Design review of the part built by this model. Coordinates are the model's own, in mm. Face numbers are marked on the shaded views. A direction names the side the tool comes from. Coordinates: 2 decimals unless noted, no trailing zeros. Loops run counter-clockwise (first coordinate to the right, second up) from the corner with the lowest first, then second, coordinate; pieces in that order, holes last.
Q1. Add section A-A on y = 23.5. Give the boundary of the cut face in (x, z).
Q2. Machinability: for the marked faces 1 and 2, which of the approach directions +Z, -Z, +X, -X, +Y, -Y give a long, thin tool a straight path to every point of the face, cutting with its end or side? Answer none if there is none.
Q3. Wall thickness on probe 1 along Y at (x, z) = (70, 10); probe 2 along Y at (x, z) = (83.5, -1); probe 3 along X at (y, z) = (21, 6): over which ranges is each line inside the solid? List them lowest first.
Q4. Add section B-B on y = 4. Give the boundary of the cut face in (x, z), and give its area (3 significant figures).
Q5. For P1, Ø2.5, axis at x = 79.77, z = 7, coming from the +Y side; P2, Ø3.5, axis at x = 70.5, z = -13, coming from the +Y side; P3, Ø5, axis at x = 58, y = 17, coming from the +Z side, all flat-tipped, find the tip position at first contact; note any pin that passes through.
```python
from build123d import *

# Parameters (mm, degrees)
SKETCH5_R             = 1.5
CUT_EXTRUDE1_DEPTH    = 4
SKETCH3_R             = 5
SKETCH3_R_2           = 2.5
BOSS_EXTRUDE3_DEPTH   = 2.5
BODY_MOVE_COPY1_ANGLE = 180
BODY_MOVE_COPY2_ANGLE = 180
BODY_MOVE_COPY3_ANGLE = 90


with BuildPart() as part:
    # Sketch1 → Revolve1 (revolve)
    with BuildSketch(Plane.XY, mode=Mode.PRIVATE) as revolve1_sk:
        with BuildLine():
            Line((33.701320748, 0), (33.701320748, 13.75))
            Line((33.701320748, 13.75), (21.201320748, 13.75))
            Line((21.201320748, 13.75), (8.201320748, 13.75))
            Line((8.201320748, 13.75), (8.201320748, 14.25))
            Line((8.201320748, 14.25), (-11.798679252, 14.25))
            Line((-11.798679252, 14.25), (-11.798679252, 13.75))
            Line((-11.798679252, 13.75), (-15.358679252, 13.75))
            ThreePointArc((-15.358679252, 13.75), (-16.23549166, 13.386812409), (-16.598679252, 12.51))
            Line((-16.598679252, 12.51), (-16.598679252, 12.5))
            Line((-16.598679252, 12.5), (-17.398679252, 12.5))
            Line((-17.398679252, 12.5), (-17.398679252, 15.00458738))
            Line((-17.398679252, 15.00458738), (-40.398679252, 15.00458738))
            Line((-40.398679252, 15.00458738), (-40.398679252, 0))
            Line((-40.398679252, 0), (33.701320748, 0))
        make_face()
    revolve(revolve1_sk.sketch.rotate(Axis((59.495632986, 0, 0), (-1, 0, 0)), 90), axis=Axis((59.495632986, 0, 0), (-1, 0, 0)))

    # Sketch5 → Cut-Extrude1 (cut)
    with BuildSketch(Plane.ZY.offset(40.398679252)):
        with Locations((-12.5, 0)):
            Circle(SKETCH5_R)
        with Locations((-10.825317547, 6.25)):
            Circle(SKETCH5_R)
        with Locations((6.25, 10.825317547)):
            Circle(SKETCH5_R)
        with Locations((12.5, 0)):
            Circle(SKETCH5_R)
        with Locations((10.825317547, -6.25)):
            Circle(SKETCH5_R)
        with Locations((6.25, -10.825317547)):
            Circle(SKETCH5_R)
    extrude(amount=-CUT_EXTRUDE1_DEPTH, mode=Mode.SUBTRACT)

    # Sketch3 → Boss-Extrude3 (add)
    with BuildSketch(Plane.ZY.offset(40.398679252)):
        with Locations((0, 5.5)):
            Circle(SKETCH3_R)
        with Locations((0, 5.5)):
            Circle(SKETCH3_R_2, mode=Mode.SUBTRACT)
    extrude(amount=BOSS_EXTRUDE3_DEPTH)


with BuildPart() as part_1:
    # Body-Move/Copy1: moved
    add(part.part.moved(Location((0, 0, 0))).rotate(Axis((-4.598679252, 0, 0), (0, 0, 1)), BODY_MOVE_COPY1_ANGLE))


with BuildPart() as part_2:
    # Body-Move/Copy2: moved
    add(part_1.part.moved(Location((0, 0, 0))).rotate(Axis((-4.598679252, 0, 0), (1.0345263845412585e-14, -0.03535860277253268, 0.9993746890981252)), BODY_MOVE_COPY2_ANGLE))


with BuildPart() as part_3:
    # Body-Move/Copy3: moved
    add(part_2.part.rotate(Axis((-4.598679252, 0, 0), (0, 0, -1)), BODY_MOVE_COPY3_ANGLE))


with BuildPart() as part_4:
    # Body-Move/Copy4: moved
    add(part_3.part.moved(Location((74.015049938, 0, 0))))


solid = part_4.part
```
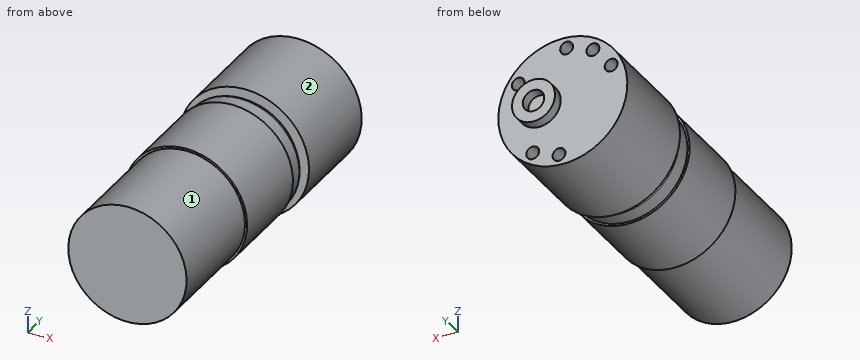
Entries:
1. outline: circle Ø30.01 at (69.42, 0)
2. face 1: -Y
2. face 2: +Y, -Y
3. probe 1: y = -38.3 to 35.8
3. probe 2: y = -12.8 to 7.2, 12.8 to 35.8
3. probe 3: x = 55.66 to 83.17
4. outline: circle Ø28.5 at (69.42, 0)
4. area: 638 mm2
5. P1: stops at y = 31.8
5. P2: stops at y = 35.8
5. P3: stops at z = 12.07
